from build123d import *

# Parameters (mm, degrees)
SKETCH_1_W          = 68
SKETCH_1_H          = 13
EXTRUDE_1_DEPTH     = 77
SKETCH_2_W          = 60
SKETCH_2_H          = 22
CUT_EXTRUDE_1_DEPTH = 10.15
FILLET_1_R          = 5
SKETCH_3_W          = 17
SKETCH_3_H          = 46
CUT_EXTRUDE_2_DEPTH = 5.2
FILLET_2_R          = 3
SKETCH_5_R          = 2.1
CUT_EXTRUDE_4_DEPTH = 4.6


with BuildPart() as part:
    # 草图1 → 凸台-拉伸1 (new body)
    with BuildSketch(Plane.YZ):
        with Locations((34, 6.5)):
            Rectangle(SKETCH_1_W, SKETCH_1_H)
    extrude(amount=EXTRUDE_1_DEPTH)

    # 草图2 → 切除-拉伸1 (cut)
    with BuildSketch(Plane.XY.offset(13)):
        with Locations((38.5, 11)):
            Rectangle(SKETCH_2_W, SKETCH_2_H)
    extrude(amount=-CUT_EXTRUDE_1_DEPTH, mode=Mode.SUBTRACT)

    # 圆角1
    fillet_1_edges = [part.edges().sort_by_distance(p)[0] for p in [
        (77, 68, 6.5),
        (77, 0, 6.5),
        (0, 68, 6.5),
        (0, 0, 6.5),
    ]]
    fillet(fillet_1_edges, radius=FILLET_1_R)

    # 草图3 → 切除-拉伸2 (cut)
    with BuildSketch(Plane.XY.offset(13)):
        with Locations((38.5, 45)):
            Rectangle(SKETCH_3_W, SKETCH_3_H)
    extrude(amount=-CUT_EXTRUDE_2_DEPTH, mode=Mode.SUBTRACT)

    # 圆角2
    fillet_2_edges = [part.edges().sort_by_distance(p)[0] for p in [
        (8.5, 22, 7.925),
        (68.5, 22, 7.925),
        (30, 22, 10.4),
        (30, 68, 10.4),
        (47, 68, 10.4),
        (47, 22, 10.4),
    ]]
    fillet(fillet_2_edges, radius=FILLET_2_R)

    # 草图5 → 切除-拉伸4 (cut)
    with BuildSketch(Plane.XY.offset(2.85)):
        with Locations((63.5, 5)):
            Circle(SKETCH_5_R)
        with Locations((13.5, 5)):
            Circle(SKETCH_5_R)
        with Locations((13.5, 19)):
            Circle(SKETCH_5_R)
        with Locations((63.5, 19)):
            Circle(SKETCH_5_R)
    extrude(amount=-CUT_EXTRUDE_4_DEPTH, mode=Mode.SUBTRACT)


solid = part.part
Verification items for the finished model (mm, model axes). A direction names the side the tool comes from. Coordinates: 2 decimals unless noted, no trailing zeros. Order: outer loops, then holes, each group sorted by start corner. A loop starts at its lowest first (then second) coordinate and runs counter-clockwise, first axis right, second up. Notation, with made-up numbers: M 29.5,39 L 49.5,39 A23 ccw 49.5,64 Z; hole C -32.75,40 d6. An arc over 180 degrees is marked long. One line per item, written item: value. Start each with the question number.
Item 1: Sectioned sample at D-D on x = 44. Record the cut outline in (y, z), then the cut area to 4 significant figures.
Item 2: Mould release check, pull along X, two halves, no side actions. Record for faces 5 (the cylindrical face through (11.952, 20.419, 1.445)), 6 (the flat face through (38, 68, 6)), 7 (the cylindrical face through (2, 1, 7)), 8 (the flat face through (38, 45, 7.8)): pulls with the +X half, pulls with the -X half, needs draft (parallel to the pull), parting line crosses it, or undercut.
Item 3: Sectioned sample at B-B on z = 10.5. Record the cut outline in (x, y), then the cut area to 3 significant figures.
Item 4: Access from +Z, -Z, +X, -X, +Y, -Y to the whole of each face (thin tool, end or side, straight path). Record for faces 1 (the cylindrical face through (76, 66, 7)), 2 (the flat face through (47, 45, 10)), 3 (the cylindrical face through (47.9, 67.14, 10.36)), 4 (the flat face through (38, 11, 2.85)).
Item 5: Depth check by flat-ended pin: P1, Ø1, axis at x = 57, y = 8, coming from the +Z side; P2, Ø1.5, axis at x = 62.5, z = 10.5, coming from the -Y side. Enter the tip coordinate at first touch or a pass-through.
Item 6: Sectioned sample at C-C on y = 26. Record the cut outline in (x, z).
Item 7: Sectioned sample at A-A on x = 13.5. Record the cut outline in (y, z).
Item 8: Thickness scan on probe 1 along Y at (x, z) = (13.5, 0.95); probe 2 along Y at (x, z) = (58, 4); probe 3 along X at (y, z) = (20.5, 3). Record the ranges inside material, lowest first.
Calculated:
1. outline: M 0,0 L 68,0 L 68,7.8 L 22,7.8 L 22,2.85 L 0,2.85 Z
1. area: 421.5 mm^2
2. face 5: undercut
2. face 6: needs draft
2. face 7: pulls with the -X half
2. face 8: undercut
3. outline: M 0,5 A5 ccw 5,0 L 8.5,0 L 8.5,19 A3 cw 11.5,22 L 27,22 A3 ccw 30,25 L 30,65 A3 ccw 27,68 L 5,68 A5 ccw 0,63 Z; M 47,25 A3 ccw 50,22 L 65.5,22 A3 cw 68.5,19 L 68.5,0 L 72,0 A5 ccw 77,5 L 77,63 A5 ccw 72,68 L 50,68 A3 ccw 47,65 Z
3. area: 3,110 mm^2
4. face 1: +Z, -Z, +X, +Y
4. face 2: +Z, +Y, -Y
4. face 3: +Z, +Y
4. face 4: +Z, -Y
5. P1: z = 2.85
5. P2: y = 22
6. outline: M 0,0 L 77,0 L 77,13 L 47,13 L 47,7.8 L 30,7.8 L 30,13 L 0,13 Z
7. outline: M 0,0 L 2.9,0 L 2.9,2.85 L 0,2.85 Z; M 7.1,0 L 16.9,0 L 16.9,2.85 L 7.1,2.85 Z; M 21.1,0 L 68,0 L 68,13 L 22,13 L 22,2.85 L 21.1,2.85 Z
8. probe 1: 0 to 2.9, 7.1 to 16.9, 21.1 to 68
8. probe 2: 22 to 68
8. probe 3: 0 to 8.9, 68.1 to 77
